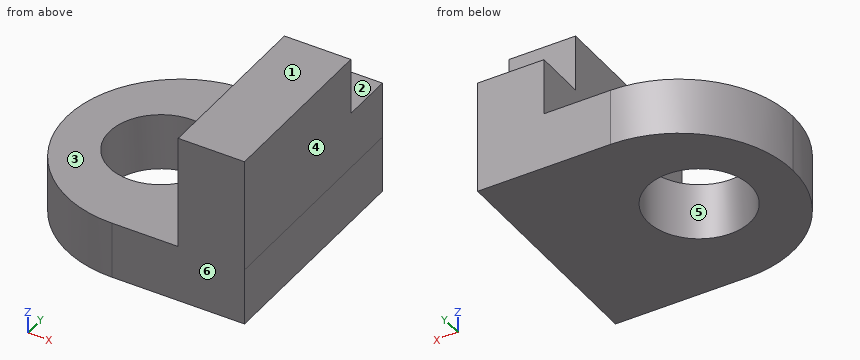
from build123d import *

# Parameters (mm, degrees)
F1_DEPTH = 25.4
F2_R     = 22.963288
F3_DEPTH = 25.401
F4_W     = 29.611313
F4_H     = 101.6
F5_DEPTH = 25.4
F6_W     = 29.611313
F6_H     = 78.306478
F7_DEPTH = 25.4


with BuildPart() as f1:
    # F0 (on Top) → F1 (new body)
    with BuildSketch(Plane.XY):
        with BuildLine():
            Line((-4.211313, -50.8), (55.011313, -50.8))
            Line((55.011313, -50.8), (55.011313, 50.8))
            Line((55.011313, 50.8), (-4.211313, 50.8))
            ThreePointArc((-4.211313, 50.8), (-40.132338, 35.921024), (-55.011313, 0))
            ThreePointArc((-55.011313, 0), (-40.132338, -35.921024), (-4.211313, -50.8))
        make_face()
    extrude(amount=F1_DEPTH)

    # F2 (on face) → F3 (cut, through all)
    with BuildSketch(Plane.XY.offset(25.4)):
        with Locations((-13.065578, 0)):
            Circle(F2_R)
    extrude(amount=-F3_DEPTH, mode=Mode.SUBTRACT)

    # F4 (on face) → F5 (join)
    with BuildSketch(Plane.XY.offset(25.4)):
        with Locations((40.205656, 0)):
            Rectangle(F4_W, F4_H)
    extrude(amount=F5_DEPTH)

    # F6 (on face) → F7 (join)
    with BuildSketch(Plane.XY.offset(50.8)):
        with Locations((40.205656, -11.646761)):
            Rectangle(F6_W, F6_H)
    extrude(amount=F7_DEPTH)


solid = f1.part
For this review, take the finished solid that the model builds, in its own axes (mm). Face numbers are marked on the shaded views. A direction names the side the tool comes from. Round coordinates to 2 decimals unless told otherwise and drop trailing zeros. Order: outer loops, then holes, each group sorted by start corner. A loop starts at its lowest first (then second) coordinate and runs counter-clockwise, first axis right, second up. Notation, with made-up numbers: M -2.75,89.5 L 46.25,89.5 A16 cw 46.25,110.5 Z; hole C 16,57.25 d9. An arc over 180 degrees is marked long. Write each question's results on one line, items separated by ' | '. Start each with the question number.
1. Add section C-C (x = -8.5). State the section outline as (y, z) points, then the cut area to 3 significant figures.
2. Draft analysis for pull direction Y (two halves, no side actions). For the marked faces 4, 5 and 6, state which applies: pulls with the +Y half, pulls with the -Y half, needs draft (parallel to the pull), parting line crosses it, or undercut.
3. To check wall thickness, follow L1, parallel to Z at x = 8.5, y = 29; L2, parallel to X at y = -23, z = 69.5; L3, parallel to Y at x = 50.5, z = 69. State the ranges of each line that lie inside material, in increasing order. Write a range as [from, to].
4. Add section D-D (y = -35). State the section outline as (x, z) points.
5. Add section A-A (y = -3). State the section outline as (x, z) points, then the cut area to 3 significant figures.
6. Clearance check with flat-ended pins moving along their axes: pin 1 Ø1.5 at (y, z) = (-30, 59.5) entering from -X; pin 2 Ø7.5 at (x, z) = (45.5, 58.5) entering from +Y. State where each tip first meets the part, or that it passes through.
7. Add section B-B (z = 17). State the section outline as (x, y) points, then the cut area to 3 significant figures.
8. Tool access review of the marked faces 1, 2 and 3: name each direction out of +Z, -Z, +X, -X, +Y, -Y from which nothing blocks a thin tool from reaching the whole face with its end or side.
Output values:
1) outline: M -50.62,0 L -22.5,0 L -22.5,25.4 L -50.62,25.4 Z; M 22.5,0 L 50.62,0 L 50.62,25.4 L 22.5,25.4 Z | area: 1,430 mm^2
2) face 4: needs draft | face 5: undercut | face 6: pulls with the -Y half
3) L1: [0, 25.4] | L2: [25.4, 55.01] | L3: [-50.8, 27.51]
4) outline: M -41.03,0 L 55.01,0 L 55.01,76.2 L 25.4,76.2 L 25.4,25.4 L -41.03,25.4 Z
5) outline: M -54.92,0 L -35.83,0 L -35.83,25.4 L -54.92,25.4 Z; M 9.7,0 L 55.01,0 L 55.01,76.2 L 25.4,76.2 L 25.4,25.4 L 9.7,25.4 Z | area: 3,140 mm^2
6) pin 1: x = 25.4 | pin 2: y = 27.51
7) outline: M -4.21,-50.8 L 55.01,-50.8 L 55.01,50.8 L -4.21,50.8 A50.8 ccw Z; hole C -13.07,0 d45.93 | area: 8,410 mm^2
8) face 1: +Z, +X, -X, +Y, -Y | face 2: +Z, +X, -X, +Y | face 3: +Z, -X, +Y, -Y
